The drawing under review shows one solid part. Ordinate dimensions are in mm from its lowest x, y, z. Round coordinates to 2 decimals unless told otherwise and drop trailing zeros. Order: outer loops, then holes, each group sorted by start corner. A loop starts at its lowest first (then second) coordinate and runs counter-clockwise, first axis right, second up. Notation, with made-up numbers: M 10,-2.5 L 26,-2.5 A17 ccw 26,14.5 Z; hole C 51,28.5 d2. An arc over 180 degrees is marked long. Answer in a Markdown table with one row per item. Add a question column.
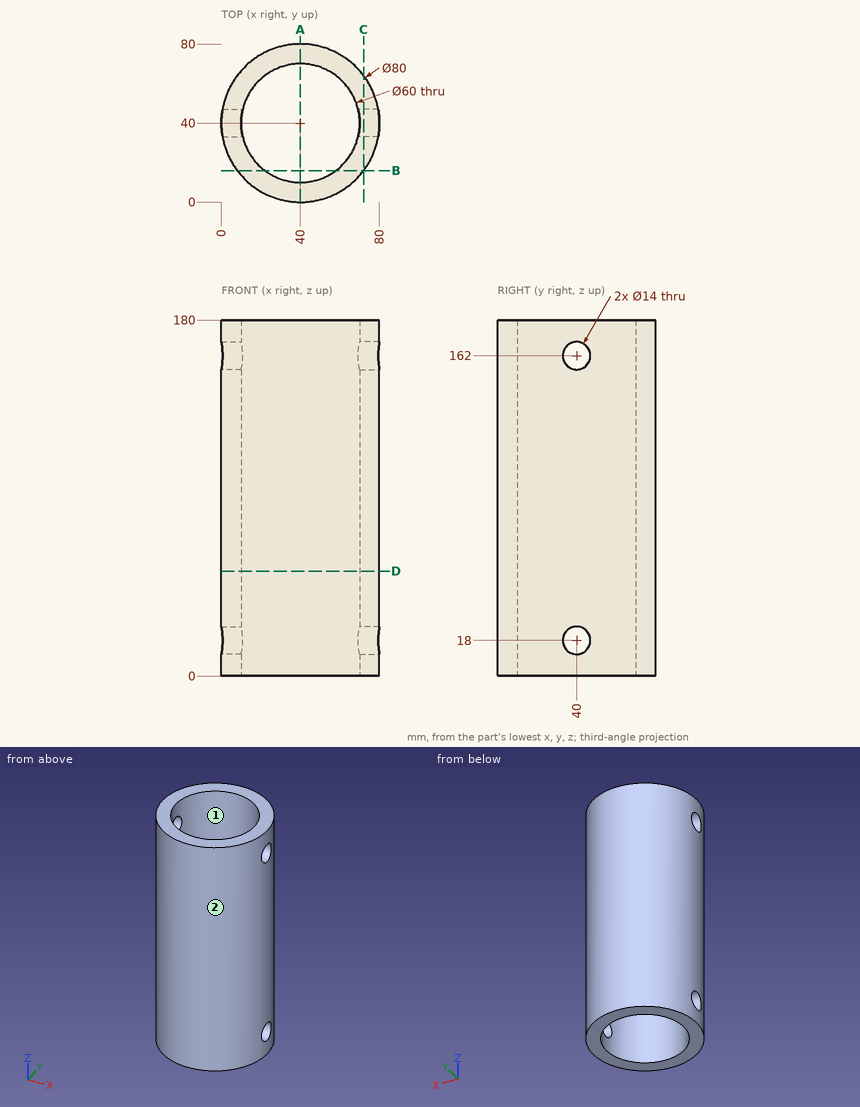
1. Consider section A-A on x = 40. Write out the cut boundary in (y, z).
2. Consider section D-D on z = 53. Write out the cut boundary in (x, y), plus the area to 3 significant figures.
3. To check wall thickness, follow probe 1 along X at (y, z) = (39, 149); probe 2 along Y at (x, z) = (40, 37); probe 3 along Y at (x, z) = (15.5, 13.5). State the ranges of each line that lie inside material, in increasing order. Write a range as [from, to].
4. Consider section C-C on x = 72. Write out the cut boundary in (y, z), plus the area to 3 significant figures.
5. Clearance check with flat-ended pins moving along their axes: pin 1 Ø1 at (x, z) = (61.5, 92) entering from -Y; pin 2 Ø10 at (y, z) = (60, 25) entering from +X; pin 3 Ø1 at (x, z) = (58.5, 159) entering from -Y; pin 4 Ø18 at (y, z) = (40, 18) entering from +X. State where each tip first meets the part, or that it passes through.
6. Consider section B-B on y = 16. Write out the cut boundary in (x, z).
7. The part is to be moulded in two halves that separate along Y. For the marked faces 1 and 2, say which applies: pulls with the +Y half, pulls with the -Y half, needs draft (parallel to the pull), parting line crosses it, or undercut.
Solved:
| question | item | result |
|---|---|---|
| 1 | outline | M 0,0 L 10,0 L 10,180 L 0,180 Z; M 70,0 L 80,0 L 80,180 L 70,180 Z |
| 2 | outline | C 40,40 d80; hole C 40,40 d60 |
| 2 | area | 2,200 mm^2 |
| 3 | probe 1 | x = [0.01, 10.02], [69.98, 79.99] |
| 3 | probe 2 | y = [0, 10], [70, 80] |
| 3 | probe 3 | y = [8.38, 22.69], [57.31, 71.62] |
| 4 | outline | M 16,0 L 64,0 L 64,180 L 16,180 Z; hole C 40,18 d14; hole C 40,162 d14 |
| 4 | area | 8,330 mm^2 |
| 5 | pin 1 | stops at y = 5.96 |
| 5 | pin 2 | stops at x = 77.08 |
| 5 | pin 3 | stops at y = 4.28 |
| 5 | pin 4 | stops at x = 80 |
| 6 | outline | M 8,0 L 22,0 L 22,180 L 8,180 Z; M 58,0 L 72,0 L 72,180 L 58,180 Z |
| 7 | face 1 | undercut |
| 7 | face 2 | parting line crosses it |
